Autodesk Inventor part; units mm, degrees
ref_plane "YZ Plane" through (0, 0, 0) normal (1, 0, 0) x (0, 1, 0)
ref_plane "XZ Plane" through (0, 0, 0) normal (0, 1, 0) x (-1, 0, 0)
ref_plane "XY Plane" through (0, 0, 0) normal (0, 0, 1) x (1, 0, 0)
sketch "Эскиз1" plane through (0, 0, 0) normal (0, 1, 0) x (-1, 0, 0)
  line L0 (0, 0) -> (13, 0)
  line L1 (13, 0) -> (13, -27.5)
  line L2 (13, -27.5) -> (0, -27.5)
  line L3 (0, -27.5) -> (0, 0)
  line L4 (11, -2) -> (6.8333, -2)
  line L5 (6.8333, -2) -> (6.8333, -6.1667)
  line L6 (6.8333, -6.1667) -> (11, -6.1667)
  line L7 (11, -6.1667) -> (11, -2)
  line L8 (11, -6.8333) -> (6.8333, -6.8333)
  line L9 (6.8333, -6.8333) -> (6.8333, -11)
  line L10 (6.8333, -11) -> (11, -11)
  line L11 (11, -11) -> (11, -6.8333)
  line L12 (11, -11.6667) -> (6.8333, -11.6667)
  line L13 (6.8333, -11.6667) -> (6.8333, -15.8333)
  line L14 (6.8333, -15.8333) -> (11, -15.8333)
  line L15 (11, -15.8333) -> (11, -11.6667)
  line L16 (11, -16.5) -> (6.8333, -16.5)
  line L17 (6.8333, -16.5) -> (6.8333, -25.5)
  line L18 (6.8333, -25.5) -> (11, -25.5)
  line L19 (11, -25.5) -> (11, -16.5)
  line L20 (6.1667, -16.5) -> (2, -16.5)
  line L21 (2, -16.5) -> (2, -20.6667)
  line L22 (2, -20.6667) -> (6.1667, -20.6667)
  line L23 (6.1667, -20.6667) -> (6.1667, -16.5)
  line L24 (6.1667, -21.3333) -> (2, -21.3333)
  line L25 (2, -21.3333) -> (2, -25.5)
  line L26 (2, -25.5) -> (6.1667, -25.5)
  line L27 (6.1667, -25.5) -> (6.1667, -21.3333)
  line L28 (6.1667, -2) -> (2, -2)
  line L29 (2, -2) -> (2, -15.8333)
  line L30 (2, -15.8333) -> (6.1667, -15.8333)
  line L31 (6.1667, -15.8333) -> (6.1667, -2)
  line L32 (8.9167, -6.1667) -> (8.9167, -6.8333)
  line L33 (8.9167, -11) -> (8.9167, -11.6667)
  line L34 (8.9167, -15.8333) -> (8.9167, -16.5)
  line L35 (4.0833, -15.8333) -> (4.0833, -16.5)
  line L36 (4.0833, -20.6667) -> (4.0833, -21.3333)
  line L37 (8.9167, -2) -> (8.9167, 0)
  line L38 (8.9167, -25.5) -> (8.9167, -27.5)
  line L39 (11, -8.9167) -> (13, -8.9167)
  line L40 (2, -8.9167) -> (0, -8.9167)
  line L41 (6.8333, -8.9167) -> (6.1667, -8.9167)
  dimension "d0" = 13
  dimension "d1" = 27.5
  dimension "d9" = 2
extrude "Выдавливание1" add sketch "Эскиз1" along normal blind 1 contours L0 L37 L4 L5 L6 L32 L8 L9 L41 L31 L28 L29 L40 L3 | L0 L1 L39 L11 L8 L32 L6 L7 L4 L37 | L40 L29 L30 L31 L41 L9 L10 L33 L12 L13 L14 L34 L16 L17 L18 L38 L2 L3 | L1 L2 L38 L18 L19 L16 L34 L14 L15 L12 L33 L10 L11 L39
sketch "Эскиз2" plane through (0, 0, 0) normal (0, -1, 0) x (1, 0, 0)
  line L0 (0, 0) -> (0, -27.5)
  line L1 (-13, 0) -> (0, 0)
  line L2 (-13, -27.5) -> (-13, 0)
  line L3 (0, -27.5) -> (-13, -27.5)
  line L4 (-6.1667, -15.8333) -> (-2, -15.8333)
  line L5 (-6.1667, -2) -> (-6.1667, -15.8333)
  line L6 (-2, -2) -> (-6.1667, -2)
  line L7 (-2, -15.8333) -> (-2, -2)
  line L8 (-2, -25.5) -> (-2, -21.3333)
  line L9 (-6.1667, -25.5) -> (-2, -25.5)
  line L10 (-6.1667, -21.3333) -> (-6.1667, -25.5)
  line L11 (-2, -21.3333) -> (-6.1667, -21.3333)
  line L12 (-6.8333, -11.6667) -> (-11, -11.6667)
  line L13 (-6.8333, -15.8333) -> (-6.8333, -11.6667)
  line L14 (-11, -15.8333) -> (-6.8333, -15.8333)
  line L15 (-11, -11.6667) -> (-11, -15.8333)
  line L16 (-11, -16.5) -> (-11, -25.5)
  line L17 (-6.8333, -16.5) -> (-11, -16.5)
  line L18 (-6.8333, -25.5) -> (-6.8333, -16.5)
  line L19 (-11, -25.5) -> (-6.8333, -25.5)
  line L20 (-11, -11) -> (-6.8333, -11)
  line L21 (-11, -6.8333) -> (-11, -11)
  line L22 (-6.8333, -6.8333) -> (-11, -6.8333)
  line L23 (-6.8333, -11) -> (-6.8333, -6.8333)
  line L24 (-11, -2) -> (-11, -6.1667)
  line L25 (-6.8333, -2) -> (-11, -2)
  line L26 (-6.8333, -6.1667) -> (-6.8333, -2)
  line L27 (-11, -6.1667) -> (-6.8333, -6.1667)
  line L28 (-2, -20.6667) -> (-2, -16.5)
  line L29 (-6.1667, -20.6667) -> (-2, -20.6667)
  line L30 (-6.1667, -16.5) -> (-6.1667, -20.6667)
  line L31 (-2, -16.5) -> (-6.1667, -16.5)
extrude "Выдавливание2" add sketch "Эскиз2" along normal blind 1 contours L0 L3 L2 L1 | L5 L6 L7 L4 | L9 L10 L11 L8 | L13 L14 L15 L12 | L17 L18 L19 L16 | L21 L22 L23 L20 | L25 L26 L27 L24 | L29 L30 L31 L28
sketch "Эскиз3" plane through (-13, 1, 0) normal (0, 0, 1) x (1, 0, 0)
  line L0 (0, -2) -> (13, -2)
  line L1 (13, -2) -> (13, -1)
  line L2 (13, -1) -> (0, -1)
  line L3 (0, -1) -> (0, -2)
  line L4 (13, -2) -> (13, 0)
  line L5 (0, -2) -> (0, 0)
  line L6 (13, -2) -> (0, -2)
  dimension "d14" = 1
extrude "Выдавливание3" add sketch "Эскиз3" along normal blind 1
sketch "Эскиз4" plane through (0, 1, -27.5) normal (0, 0, -1) x (-1, 0, 0)
  line L0 (6.8333, -1) -> (11, -1)
  line L1 (13, -2) -> (0, -2)
  line L2 (0, -2) -> (0, -1)
  line L3 (0, -1) -> (13, -1)
  line L4 (13, -1) -> (13, -2)
extrude "Выдавливание4" add sketch "Эскиз4" along normal blind 1
properties part number "Лого ШП"
Read the model definition and answer for the solid it produces. Units are mm, in the model's axes. A direction names the side the tool comes from. Give positions to 0.01 mm unless a question says otherwise; leave off trailing zeros. Write each loop counter-clockwise with the first axis right and the second up, starting at its lowest first coordinate (ties: lowest second). Pieces come first, ordered by that corner, then holes. Notation, with made-up numbers: (65, 24) -> (89, 24) arc R16 ccw to (89, 35) -> close; hole circle Ø6 at (84, -35). An arc over 180 degrees is marked (long way). Answer as a JSON object with one key per item and string values. Group by question number.
1) A tool of negligible diameter and unlimited length cuts with its end or side. For faces 1 (the flat face through (-8.9, 0.5, -25.5)), 2 (the flat face through (-6.4, 1, -13.6)), from which of +Z, -Z, +X, -X, +Y, -Y can it reach the whole face along a straight path? Write none if from no direction.
2) Consider L1, parallel to X at y = 0.45, z = -21.5; L2, parallel to Z at x = -10.75, y = 0.3; L3, parallel to Z at x = -3.75, y = 0.8. Determine where each line is inside the solid, lowest interval first. Write a range as from..to.
3) Find section B-B (y = 0.65). Count the separate pieces of the cut face and the enclosed holes in it, and give its area (3 significant figures).
4) The mould has two halves that part along X. Classify faces 3 (the flat face through (-6, 0, -28)), 4 (the flat face through (0, 0, -14)), 5 (the flat face through (-8.9, 0.5, -2)): +X half, -X half, draft (parallel to the pull), parting line (faces both ways), or undercut.
5) Find section A-A (x = -4.25). Write down the section's boundary in (y, z), and give its area (3 significant figures).
6) Each of these flat-tipped pins is pushed along its axis until it touches: P1, Ø3.5, axis at x = -9, z = -14.5, coming from the +Y side; P2, Ø0.8, axis at x = -5, y = 0.5, coming from the +Z side; P3, Ø0.5, axis at x = -9, y = 0.5, coming from the -Z side; P4, Ø2, axis at x = -9.5, z = -9.5, coming from the +Y side. Where does it stop, or does it pass through?
7) Find section D-D (x = -11.75). Write down the section's boundary in (y, z), and give its area (3 significant figures).
8) Find section C-C (z = -4). Write down the section's boundary in (x, y).
Values follow:
{
 "1": {"face 1": "+Y", "face 2": "+Z, -Z, +X, -X, +Y"},
 "2": {"L1": "x = -13..-11, -6.83..-6.17, -2..0", "L2": "z = -27.5..-25.5, -16.5..-15.83, -11.67..-11, -6.83..-6.17, -2..0", "L3": "z = -27.5..-25.5, -21.33..-20.67, -16.5..-15.83, -2..0"},
 "3": {"separate pieces": "1", "enclosed holes": "7", "area": "176 mm2"},
 "4": {"face 3": "draft", "face 4": "+X half", "face 5": "undercut"},
 "5": {"outline": "(-1, -28.5) -> (0, -28.5) -> (0, -27.5) -> (1, -27.5) -> (1, -25.5) -> (0, -25.5) -> (0, -21.33) -> (1, -21.33) -> (1, -20.67) -> (0, -20.67) -> (0, -16.5) -> (1, -16.5) -> (1, -15.83) -> (0, -15.83) -> (0, -2) -> (1, -2) -> (1, 0) -> (0, 0) -> (0, 1) -> (-1, 1) -> close", "area": "34.8 mm2"},
 "6": {"P1": "stops at y = 1", "P2": "stops at z = 0", "P3": "stops at z = -27.5", "P4": "stops at y = 0"},
 "7": {"outline": "(-1, -28.5) -> (0, -28.5) -> (0, -27.5) -> (1, -27.5) -> (1, 0) -> (0, 0) -> (0, 1) -> (-1, 1) -> close", "area": "57.0 mm2"},
 "8": {"outline": "(-13, -1) -> (0, -1) -> (0, 1) -> (-2, 1) -> (-2, 0) -> (-6.17, 0) -> (-6.17, 1) -> (-6.83, 1) -> (-6.83, 0) -> (-11, 0) -> (-11, 1) -> (-13, 1) -> close"}
}
